```python
from build123d import *

# Parameters (mm, degrees)
F0_W     = 86
F0_H     = 152
F0_W_2   = 50
F0_H_2   = 8
F1_DEPTH = 12
F2_DEPTH = 31
F3_R     = 7


with BuildPart() as f1:
    # F0 (on Top) → F1 (new body)
    with BuildSketch(Plane.XY):
        Rectangle(F0_W, F0_H)
        with Locations((0, -60.848527)):
            Rectangle(F0_W_2, F0_H_2, mode=Mode.SUBTRACT)
        Polygon((-29.75, -50), (-29.75, 50), (9.75, 50), (9.75, 55), (29.75, 55), (29.75, 50), (35.75, 50), (35.75, 10), (29.75, 10), (29.75, -50), (29.75, -55), (9.75, -55), (9.75, -50), align=None, mode=Mode.SUBTRACT)
        with Locations((0, 60.848527)):
            Rectangle(F0_W_2, F0_H_2, mode=Mode.SUBTRACT)
    extrude(amount=F1_DEPTH)

    # F0 (on Top) → F2 (join)
    with BuildSketch(Plane.XY):
        with Locations((0, 60.848527)):
            Rectangle(F0_W_2, F0_H_2)
        with Locations((0, -60.848527)):
            Rectangle(F0_W_2, F0_H_2)
    extrude(amount=F2_DEPTH)

    # F3
    f3_edges = [f1.edges().sort_by_distance(p)[0] for p in [
        (-43, -76, 6),
        (43, -76, 6),
        (43, 76, 6),
        (-43, 76, 6),
        (43, 0, 0),
        (0, -76, 0),
        (-43, 0, 0),
        (0, 76, 0),
    ]]
    fillet(f3_edges, radius=F3_R)


solid = f1.part
```
Geometry: final body of the model. Coordinates: model frame, mm. A direction names the side the tool comes from. Round coordinates to 2 decimals unless told otherwise and drop trailing zeros. Order: outer loops, then holes, each group sorted by start corner. A loop starts at its lowest first (then second) coordinate and runs counter-clockwise, first axis right, second up. Notation, with made-up numbers: M 64,19 L 73,19 A37 ccw 73,58 Z; hole C -6.5,88.5 d11. An arc over 180 degrees is marked long. One line per item, written item: value.
(1) Line query: probe 1 along Y at (x, z) = (1.5, 18); probe 2 along X at (y, z) = (-34, 11); probe 3 along Y at (x, z) = (21, 7.5). Output: solid intervals per line, ascending. Write a range as [from, to].
Result sheet:
probe 1: [-64.85, -56.85], [56.85, 64.85]
probe 2: [-43, -29.75], [29.75, 43]
probe 3: [-76, -55], [55, 76]
(2) Cut plane B-B (x = -17.5). Return the cut outline in (y, z).
Result sheet:
outline: M -76,7 A7 ccw -69,0 L -50,0 L -50,12 L -56.85,12 L -56.85,31 L -64.85,31 L -64.85,12 L -76,12 Z; M 50,0 L 69,0 A7 ccw 76,7 L 76,12 L 64.85,12 L 64.85,31 L 56.85,31 L 56.85,12 L 50,12 Z
(3) Cut plane D-D (y = -51.5). Return the cut outline in (x, z), and give its area (3 significant figures).
Result sheet:
outline: M -43,7 A7 ccw -36,0 L 9.75,0 L 9.75,12 L -43,12 Z; M 29.75,0 L 36,0 A7 ccw 43,7 L 43,12 L 29.75,12 Z
area: 771 mm2
(4) Pin query (flat end, axial travel): P1, Ø4, axis at x = 21, z = 23.5, coming from the +Y side; P2, Ø1.8, axis at x = 32.5, z = 5.5, coming from the -Y side; P3, Ø2.5, axis at y = 61.5, z = 25, coming from the -X side. Return the tip coordinate at first contact, or that it passes through.
Result sheet:
P1: y = 64.85
P2: y = -75.97
P3: x = -25
(5) Pull-direction query (Y, two-part tool) for faces 1 (the cylindrical face through (41, 1, 2.1)), 2 (the flat face through (-10, -50, 6)), 3 (the flat face through (-1, -76, 9)); classes: pulls with the +Y half, pulls with the -Y half, needs draft (parallel to the pull), parting line crosses it, or undercut.
Result sheet:
face 1: needs draft
face 2: undercut
face 3: pulls with the -Y half
(6) Reachability of faces 4 (the flat face through (-25, 61, 21)), 5 (the flat face through (0, 56.849, 21)), 6 (the flat face through (20, 55, 6)), 7 (the flat face through (25, -61, 21)) from +Z, -Z, +X, -X, +Y, -Y: full face, straight path, thin tool, end or side. Return the list, or none.
Result sheet:
face 4: +Z, -X, +Y, -Y
face 5: +Z, +X, -X
face 6: +Z, -Z
face 7: +Z, +X, +Y, -Y
(7) Cut plane C-C (z = 20.5). Return the cut outline in (x, y).
Result sheet:
outline: M -25,-64.85 L 25,-64.85 L 25,-56.85 L -25,-56.85 Z; M -25,56.85 L 25,56.85 L 25,64.85 L -25,64.85 Z
(8) Cut plane A-A (y = -21.5). Return the cut outline in (x, z), and give its area (3 significant figures).
Result sheet:
outline: M -43,7 A7 ccw -36,0 L -29.75,0 L -29.75,12 L -43,12 Z; M 29.75,0 L 36,0 A7 ccw 43,7 L 43,12 L 29.75,12 Z
area: 297 mm2
